from build123d import *

# Parameters (mm, degrees)
SKETCH_1_R          = 37
SKETCH_1_R_2        = 35
EXTRUDE_1_DEPTH     = 1
SKETCH_1_R_3        = 29.15
EXTRUDE_1_2_DEPTH   = 1
EXTRUDE_START       = 1
SKETCH_2_R          = 37
EXTRUDE_2_DEPTH     = 1
SKETCH_3_R          = 34
EXTRUDE_3_DEPTH     = 11
SKETCH_5_R          = 37
EXTRUDE_4_DEPTH     = 1
SKETCH_4_R          = 37
SKETCH_4_R_2        = 35
SKETCH_4_R_3        = 29.15
EXTRUDE_5_DEPTH     = 1
SKETCH_6_R          = 5
CUT_EXTRUDE_1_DEPTH = 55.433445601


with BuildPart() as part:
    # Sketch 1 → Extrude 1 (new body)
    with BuildSketch(Plane.XY):
        Circle(SKETCH_1_R)
        Circle(SKETCH_1_R_2, mode=Mode.SUBTRACT)
    extrude(amount=EXTRUDE_1_DEPTH)



with BuildPart() as body_2:
    # Sketch 1 → Extrude 1 2 (new body)
    with BuildSketch(Plane.XY):
        Circle(SKETCH_1_R_3)
    extrude(amount=EXTRUDE_1_2_DEPTH)


with BuildPart() as part_1:
    add(part.part)

    add(body_2.part)  # Extrude 2 merges body 2
    # Sketch 2 → Extrude 2 (add)
    with BuildSketch(Plane(origin=(0, 0, 0), x_dir=(-1, 0, 0), z_dir=(0, 0, -1)).offset(EXTRUDE_START)):
        Circle(SKETCH_2_R)
    extrude(amount=-EXTRUDE_2_DEPTH)

    # Sketch 3 → Extrude 3 (add)
    with BuildSketch(Plane(origin=(0, 0, -1), x_dir=(-1, 0, 0), z_dir=(0, 0, -1))):
        Circle(SKETCH_3_R)
    extrude(amount=EXTRUDE_3_DEPTH)

    # Sketch 5 → Extrude 4 (add)
    with BuildSketch(Plane(origin=(0, 0, -12), x_dir=(-1, 0, 0), z_dir=(0, 0, -1)).offset(EXTRUDE_START)):
        Circle(SKETCH_5_R)
    extrude(amount=-EXTRUDE_4_DEPTH)

    # Sketch 4 → Extrude 5 (add)
    # profile 1 of 2: a face of its own
    with BuildSketch(Plane(origin=(0, 0, -13), x_dir=(-1, 0, 0), z_dir=(0, 0, -1)).offset(EXTRUDE_START)):
        Circle(SKETCH_4_R)
        with Locations(Location((0, 0, 0), (0, 0, 180))):
            Circle(SKETCH_4_R_2, mode=Mode.SUBTRACT)
    # profile 2 of 2: a face of its own
    with BuildSketch(Plane(origin=(0, 0, -13), x_dir=(-1, 0, 0), z_dir=(0, 0, -1)).offset(EXTRUDE_START)):
        Circle(SKETCH_4_R_3)
    extrude(amount=-EXTRUDE_5_DEPTH)

    # Sketch 6 → Cut-Extrude 1 (cut, through all)
    with BuildSketch(Plane(origin=(0, 0, -14), x_dir=(-1, 0, 0), z_dir=(0, 0, -1))):
        Circle(SKETCH_6_R)
    extrude(amount=-CUT_EXTRUDE_1_DEPTH, mode=Mode.SUBTRACT)


solid = part_1.part
The model under review builds one solid part; all positions refer to its coordinate system, in mm. A direction names the side the tool comes from. Round coordinates to 2 decimals unless told otherwise and drop trailing zeros. Write each loop counter-clockwise with the first axis right and the second up, starting at its lowest first coordinate (ties: lowest second). Pieces come first, ordered by that corner, then holes. Notation, with made-up numbers: M 13,-18 L 62,-18 A4 cw 62,-12 Z; hole C 82.5,60 d1. An arc over 180 degrees is marked long. Use a Markdown table: item, result. Add a question column.
Q1. Machinability: for faces 1 (the face through (0, -6, 1)), 2 (the face through (-11, -33, -1)), 3 (the face through (8.02, -36.12, -13.01)), 4 (the face through (8, 29, 0)), 5 (the face through (8, 29, -13)), which of the approach directions +Z, -Z, +X, -X, +Y, -Y give a long, thin tool a straight path to every point of the face, cutting with its end or side? Answer none if there is none.
Q2. The part is to be moulded in two halves that separate along Y. For faces 6 (the face through (6.319, -28.457, -13.507)), 7 (the face through (-18.28, 28.67, -6.42)), 8 (the face through (0, -6, -14)), 9 (the face through (1.08, -4.88, -6.6)), say which applies: pulls with the +Y half, pulls with the -Y half, needs draft (parallel to the pull), parting line crosses it, or undercut.
Q3. To check wall thickness, follow line 1 (Y direction, x = 0, z = 0.5); line 2 (Z direction, x = -33, y = -12); line 3 (Y direction, x = 0, z = -5.5). State the ranges of each line that lie inside material, in increasing order.
Q4. We need section C-C, the plane z = -9.5. State the section outline as (x, y) points, plus the area to 3 significant figures.
Q5. We need section D-D, the plane y = -14.5. State the section outline as (x, z) points, plus the area to 3 significant figures.
Q6. Insertion check: pin 1 (3 mm diameter, centred on y = 28, z = -0.5, fed in from +X); pin 2 (3 mm diameter, centred on y = 5, z = -3.5, fed in from +X); pin 3 (2 mm diameter, centred on x = 23, z = -7.5, fed in from +Y). Each pin has a flat end and moves straight along its axis. Give the tip position at first contact, or say it passes through.
Findings below:
| question | item | result |
|---|---|---|
| 1 | face 1 | +Z, +X, -X, +Y, -Y |
| 1 | face 2 | none |
| 1 | face 3 | +Z, -Z |
| 1 | face 4 | +Z |
| 1 | face 5 | -Z |
| 2 | face 6 | undercut |
| 2 | face 7 | parting line crosses it |
| 2 | face 8 | needs draft |
| 2 | face 9 | undercut |
| 3 | line 1 | y = -37 to -35, -29.15 to -5, 5 to 29.15, 35 to 37 |
| 3 | line 2 | z = -14 to -12, -1 to 1 |
| 3 | line 3 | y = -34 to -5, 5 to 34 |
| 4 | outline | C 0,0 d68; hole C 0,0 d10 |
| 4 | area | 3,550 mm² |
| 5 | outline | M -34.04,-14 L -31.86,-14 L -31.86,-13 L -25.29,-13 L -25.29,-14 L 25.29,-14 L 25.29,-13 L 31.86,-13 L 31.86,-14 L 34.04,-14 L 34.04,-12 L 30.75,-12 L 30.75,-1 L 34.04,-1 L 34.04,1 L 31.86,1 L 31.86,0 L 25.29,0 L 25.29,1 L -25.29,1 L -25.29,0 L -31.86,0 L -31.86,1 L -34.04,1 L -34.04,-1 L -30.75,-1 L -30.75,-12 L -34.04,-12 Z |
| 5 | area | 923 mm² |
| 6 | pin 1 | stops at x = 25.82 |
| 6 | pin 2 | stops at x = 33.82 |
| 6 | pin 3 | stops at y = 25.92 |
